Geometry check sheet. Reference: the model listing, model coordinates, mm. A direction names the side the tool comes from. Coordinates: 2 decimals unless noted, no trailing zeros. Write each loop counter-clockwise with the first axis right and the second up, starting at its lowest first coordinate (ties: lowest second). Pieces come first, ordered by that corner, then holes. Notation, with made-up numbers: (58.5, 34) -> (110.5, 34) arc R31 ccw to (110.5, 60) -> close; hole circle Ø9 at (-4, 78.25). An arc over 180 degrees is marked (long way). Put each result on its own line as item: value. Start each with the question number.
Autodesk Inventor part; units mm, degrees
ref_plane "YZ Plane" through (0, 0, 0) normal (1, 0, 0) x (0, 1, 0)
ref_plane "XZ Plane" through (0, 0, 0) normal (0, 1, 0) x (-1, 0, 0)
ref_plane "XY Plane" through (0, 0, 0) normal (0, 0, 1) x (1, 0, 0)
sketch "Sketch1" plane through (0, 0, 0) normal (0, 0, 1) x (1, 0, 0)
  arc A0 (0, 40) -> (0, -40) centre (0, 0) ccw
  arc A1 (265, -40) -> (265, 40) centre (265, 0) ccw
  line L0 (0, 0) -> (265, 0) construction
  line L1 (0, 40) -> (265, 40)
  line L2 (0, -40) -> (265, -40)
  arc A2 (40, 0) -> (0, 40) centre (0, 0) ccw construction
  arc A3 (0, -40) -> (40, 0) centre (0, 0) ccw construction
  arc A4 (225, 0) -> (265, -40) centre (265, 0) ccw construction
  arc A5 (265, 40) -> (225, 0) centre (265, 0) ccw construction
  circle A6 centre (0, 0) radius 5
  circle A7 centre (265, 0) radius 5
  dimension "d0" = 80
  dimension "d1" = 80
  dimension "d2" = 265
  dimension "d3" = 10
  dimension "d4" = 10
extrude "Extrusion1" add sketch "Sketch1" along normal mid plane 70
sketch "Sketch2" plane through (0, 40, 35) normal (0, 1, 0) x (1, 0, 0)
  line L0 (-40, 0) -> (0, 0) construction
  line L1 (-40, 0) -> (45, 0) construction
  line L2 (45, 70) -> (45, 69.4311) construction
  line L3 (305, 70) -> (305, 0) construction
  line L4 (55, 10) -> (305, 10) construction
  line L5 (305, 10) -> (305, 60) construction
  line L6 (305, 60) -> (55, 60) construction
  line L7 (45, 60) -> (45, 10) construction
  line L8 (0, 70) -> (265, 70) construction
  line L9 (265, 0) -> (0, 0) construction
  line L10 (45, 60) -> (305, 60) construction
  line L11 (305, 60) -> (305, 70)
  line L12 (305, 70) -> (45, 70)
  line L13 (45, 70) -> (45, 60) construction
  line L14 (45, 10) -> (305, 10) construction
  line L15 (305, 10) -> (305, 0)
  line L16 (305, 0) -> (45, 0)
  line L17 (45, 0) -> (45, 0)
  line L18 (55, 60) -> (45, 70)
  line L19 (55, 10) -> (45, 0)
  line L20 (55, 60) -> (305, 60)
  line L21 (305, 10) -> (50, 10)
  line L22 (-40, 70) -> (-40, 0)
  line L23 (-40, 10) -> (40, 10)
  line L24 (40, 10) -> (40, 60)
  line L25 (40, 60) -> (-40, 60)
  line L26 (-40, 60) -> (-40, 10)
  point P0 (0, 35)
  point P1 (45, 70)
  point P2 (45, 0)
  point P3 (55, 10)
  dimension "d7" = 85
  dimension "d8" = 10
  dimension "d9" = 10
  dimension "d10" = 10
  dimension "d11" = 10
  dimension "d12" = 10
  dimension "d13" = 10
  dimension "d14" = 80
extrude "Extrusion2" cut sketch "Sketch2" against normal through all
fillet "Fillet1" radius 3 26 edges at (305, 0, 25) (160, -40, 25) (160, 40, 25) (305, 0, -25) (160, -40, -25) (160, 40, -25) (-40, 0, 35) (22.5, -40, 35) (22.5, 40, 35) (-40, 0, 25) (20, -40, 25) (20, 40, 25) (-40, 0, -25) (20, -40, -25) (20, 40, -25) (-40, 0, -35) (22.5, -40, -35) (22.5, 40, -35) (40, 40, 0) (40, -40, 0) (50, -40, 30) (50, 40, 30) (50, 40, -30) (50, -40, -30) (40, 0, -25) (40, 0, 25)
equation "\"d12\" = d10"
equation "\"d13\" = d12"
properties part number "Arm1"
Item 1: Scan lines: line 1 along Y through (x, z) = (0, -32.5); line 2 along X through (y, z) = (0, 6); line 3 along Z through (x, y) = (85, -24.5). Record each from-to range of solid material in increasing order. Write a range as [from, to].
Item 2: Go/stop test with flat-tipped pins: P1, Ø1, axis at y = 1, z = 9, coming from the -X side; P2, Ø10, axis at x = 125.5, y = -14, coming from the +Z side; P3, Ø1, axis at y = -25, z = -15, coming from the +X side. Record where each tip stops, or that it passes through.
Item 3: Section check C-C, the plane y = 0. Give the number of separate pieces and of enclosed holes in the cut face, and give its area (3 significant figures).
Item 4: Mould release check, pull along Z, two halves, no side actions. Record for faces 4 (the cylindrical face through (-1.08, 4.88, -30.07)), 5 (the flat face through (13, 1, -35)), 6 (the flat face through (9, 1, -25)): released by +Z, released by -Z, zero draft, split by the parting line, or undercut.
Item 5: Section check A-A, the plane x = 93.5. Enter the section's corners in (y, z).
Item 6: Access from +Z, -Z, +X, -X, +Y, -Y to the whole of each face (thin tool, end or side, straight path). Record for faces 1 (the flat face through (180, 1, 25)), 2 (the flat face through (8, 1, 25)), 3 (the flat face through (177, 1, -25)).
Item 7: Section check B-B, the plane z = -2. Enter the section's corners in (x, y), and give its area (3 significant figures).
From the geometry:
1. line 1: [-39.96, -5], [5, 39.96]
1. line 2: [40, 260], [270, 305]
1. line 3: [-25, 25]
2. P1: x = 40
2. P2: z = 25
2. P3: x = 296.62
3. separate pieces: 4
3. enclosed holes: 0
3. area: 14,300 mm²
4. face 4: zero draft
4. face 5: released by -Z
4. face 6: undercut
5. outline: (-40, -22) arc R3 ccw to (-37, -25) -> (37, -25) arc R3 ccw to (40, -22) -> (40, 22) arc R3 ccw to (37, 25) -> (-37, 25) arc R3 ccw to (-40, 22) -> close
6. face 1: +Z, +X, +Y, -Y
6. face 2: -X, +Y, -Y
6. face 3: -Z, +X, +Y, -Y
7. outline: (40, -37) arc R3 ccw to (43, -40) -> (265, -40) arc R40 ccw to (265, 40) -> (43, 40) arc R3 ccw to (40, 37) -> close; hole circle Ø10 at (265, 0)
7. area: 20,400 mm²
